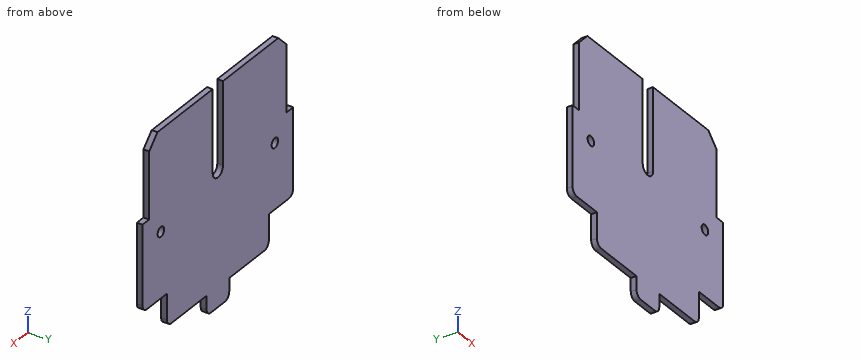
```python
from build123d import *

# Parameters (mm, degrees)
SKETCH1_R           = 1.1
BOSS_EXTRUDE1_DEPTH = 0.65


with BuildPart() as part:
    # Sketch1 → Boss-Extrude1 (new, symmetric)
    with BuildSketch(Plane(origin=(0, 0, 0), x_dir=(1, 0, 0), z_dir=(0, 1, 0))):
        with BuildLine():
            Line((20.45, -24.375), (23.25, -21.575))
            Line((23.25, -21.575), (23.25, -8.875))
            Line((23.25, -8.875), (23.25, -6.625))
            Line((23.25, -6.625), (25.5, -6.625))
            Line((25.5, -6.625), (25.5, 11.175))
            ThreePointArc((25.5, 11.175), (25.060660172, 12.235660172), (24, 12.675))
            Line((24, 12.675), (17.25, 12.675))
            Line((17.25, 12.675), (17.25, 18.425))
            ThreePointArc((17.25, 18.425), (16.810660172, 19.485660172), (15.75, 19.925))
            Line((15.75, 19.925), (3.85, 19.925))
            Line((3.85, 19.925), (3.85, 22.875))
            ThreePointArc((3.85, 22.875), (3.410660172, 23.935660172), (2.35, 24.375))
            Line((2.35, 24.375), (-2.35, 24.375))
            ThreePointArc((-2.35, 24.375), (-3.410660172, 23.935660172), (-3.85, 22.875))
            Line((-3.85, 22.875), (-3.85, 19.925))
            Line((-3.85, 19.925), (-15.75, 19.925))
            ThreePointArc((-15.75, 19.925), (-16.810660172, 19.485660172), (-17.25, 18.425))
            Line((-17.25, 18.425), (-17.25, 12.675))
            Line((-17.25, 12.675), (-24, 12.675))
            ThreePointArc((-24, 12.675), (-25.060660172, 12.235660172), (-25.5, 11.175))
            Line((-25.5, 11.175), (-25.5, -6.625))
            Line((-25.5, -6.625), (-23.25, -6.625))
            Line((-23.25, -6.625), (-23.25, -8.875))
            Line((-23.25, -8.875), (-23.25, -21.575))
            Line((-23.25, -21.575), (-20.45, -24.375))
            Line((-20.45, -24.375), (-1.75, -24.375))
            Line((-1.75, -24.375), (-1.75, -5.875))
            ThreePointArc((-1.75, -5.875), (0, -4.125), (1.75, -5.875))
            Line((1.75, -5.875), (1.75, -24.375))
            Line((1.75, -24.375), (20.45, -24.375))
        make_face()
        with Locations(Location((19.3, -1.925, 0), (0, 0, 270))):
            Circle(SKETCH1_R, mode=Mode.SUBTRACT)
        with Locations(Location((-19.3, -1.925, 0), (0, 0, 90))):
            Circle(SKETCH1_R, mode=Mode.SUBTRACT)
    extrude(amount=BOSS_EXTRUDE1_DEPTH, both=True)


solid = part.part
```
Verification items for the finished model (mm, model axes). Give positions to 0.01 mm unless a question says otherwise; leave off trailing zeros. Order: outer loops, then holes, each group sorted by start corner. A loop starts at its lowest first (then second) coordinate and runs counter-clockwise, first axis right, second up. Notation, with made-up numbers: M 54,29.25 L 72,29.25 A19 cw 72,60.25 Z; hole C 9,-32.75 d2. An arc over 180 degrees is marked long. Return JSON: item names as keys, results as strings. Group by question number.
1) Scan lines: line 1 (X direction, y = 0.1, z = 2); line 2 (Z direction, x = -19.3, y = 0.05) (3 decimals); line 3 (X direction, y = 0.5, z = 2.5). Record each from-to range of solid material in increasing order.
2) Section check D-D on x = -14.5. Record the cut outline in (y, z) (3 decimals), and give its area (3 significant figures).
3) Section check C-C on z = 15. Record the cut outline in (x, y), and give its area (3 significant figures).
4) Go/stop test with flat-tipped pins: pin 1 Ø0.6 at (x, y) = (-24.5, 0.5) entering from +Z (3 decimals); pin 2 Ø0.6 at (y, z) = (0, -15.5) entering from +X; pin 3 Ø0.6 at (x, y) = (7.5, 0) entering from -Z (3 decimals). Record where each tip stops, or that it passes through.
5) Section check B-B on y = -0.45. Give the number of separate pieces and of enclosed holes in the cut face, and give its area (3 significant figures).
6) Section check A-A on x = 19.3. Record the cut outline in (y, z) (3 decimals).
Answer block:
{
 "1": {"line 1": "x = -25.5 to -20.4, -18.2 to 18.2, 20.4 to 25.5", "line 2": "z = -12.675 to 0.825, 3.025 to 24.375", "line 3": "x = -25.5 to -20.24, -18.36 to 18.36, 20.24 to 25.5"},
 "2": {"outline": "M -0.65,-19.925 L 0.65,-19.925 L 0.65,24.375 L -0.65,24.375 Z", "area": "57.6 mm^2"},
 "3": {"outline": "M -23.25,-0.65 L -1.75,-0.65 L -1.75,0.65 L -23.25,0.65 Z; M 1.75,-0.65 L 23.25,-0.65 L 23.25,0.65 L 1.75,0.65 Z", "area": "55.9 mm^2"},
 "4": {"pin 1": "stops at z = 6.625", "pin 2": "stops at x = 17.25", "pin 3": "stops at z = -19.925"},
 "5": {"separate pieces": "1", "enclosed holes": "2", "area": "2,010 mm^2"},
 "6": {"outline": "M -0.65,-12.675 L 0.65,-12.675 L 0.65,0.825 L -0.65,0.825 Z; M -0.65,3.025 L 0.65,3.025 L 0.65,24.375 L -0.65,24.375 Z"}
}
